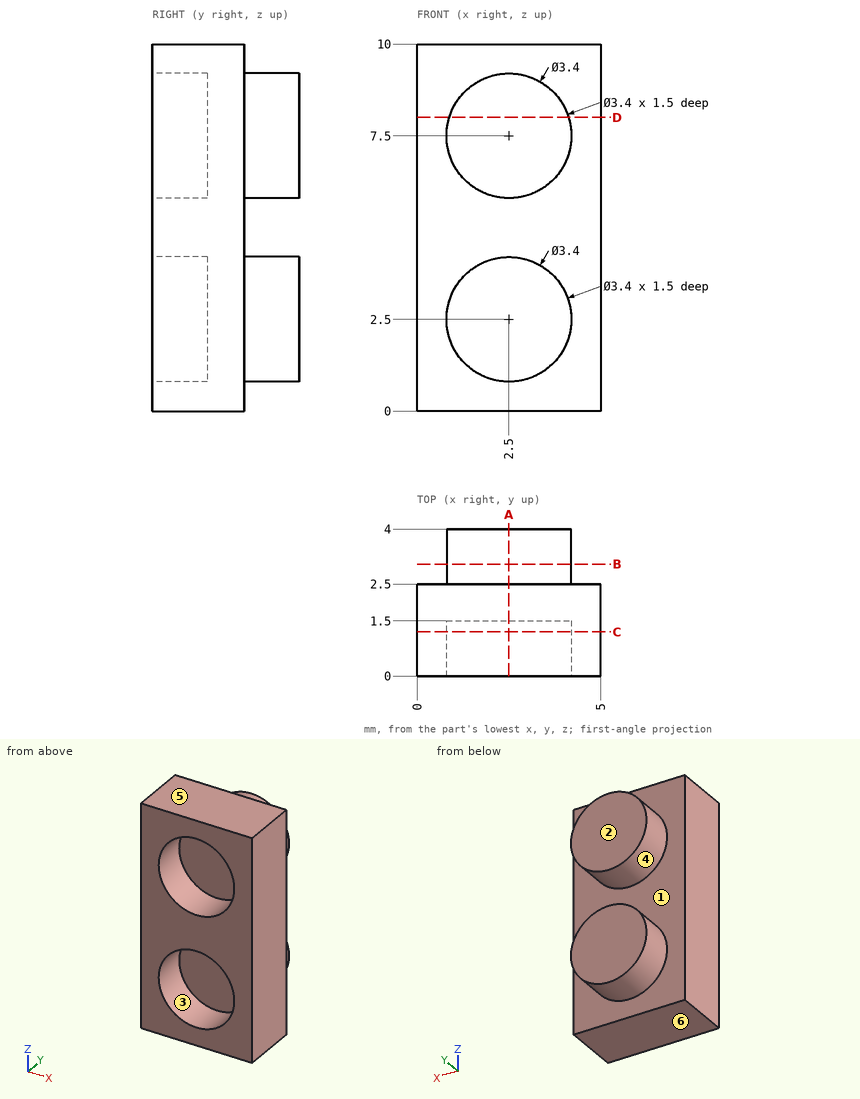
Verification items for this drawing (mm, ordinates from the low corner). A direction names the side the tool comes from. Round coordinates to 2 decimals unless told otherwise and drop trailing zeros. Order: outer loops, then holes, each group sorted by start corner. A loop starts at its lowest first (then second) coordinate and runs counter-clockwise, first axis right, second up. Notation, with made-up numbers: (69, 0.25) - (76, 0.25) arc R20 ccw to (76, 19.25) - close; hole circle Ø10 at (-37.5, 31). An arc over 180 degrees is marked (long way). Use CSV: the item, a comma, the result in double quotes. Start each with the question number.
1) Mould release check, pull along Z, two halves, no side actions. Record for the marked faces 4, 5 and 6: +Z half, -Z half, draft (parallel to the pull), parting line (faces both ways), or undercut.
2) Go/stop test with a flat-tipped pin: P1, Ø2, axis at x = 2.5, z = 8, coming from the -Y side. Record where the tip stops, or that it passes through.
3) Thickness scan on L1, parallel to Z at x = 2.5, y = 0.8; L2, parallel to Y at x = 1.75, z = 3.5; L3, parallel to Y at x = 4.5, z = 9.75. Record the ranges inside material, lowest first.
4) Access from +Z, -Z, +X, -X, +Y, -Y to the whole of each face (thin tool, end or side, straight path). Record for the marked faces 1, 2 and 3.
5) Section check D-D, the plane z = 8. Record the cut outline in (x, y).
6) Section check A-A, the plane x = 2.5. Record the cut outline in (y, z).
7) Section check C-C, the plane y = 1.2. Record the cut outline in (x, z), plus the area to 3 significant figures.
8) Section check B-B, the plane y = 3.05. Record the cut outline in (x, z), plus the area to 3 significant figures.
Answers:
1,face 4,"undercut"
1,face 5,"+Z half"
1,face 6,"-Z half"
2,P1,"stops at y = 1.5"
3,L1,"z = 0 to 0.8, 4.2 to 5.8, 9.2 to 10"
3,L2,"y = 1.5 to 4"
3,L3,"y = 0 to 2.5"
4,face 1,"+Y"
4,face 2,"+Z, -Z, +X, -X, +Y"
4,face 3,"-Y"
5,outline,"(0, 0) - (0.88, 0) - (0.88, 1.5) - (4.12, 1.5) - (4.12, 0) - (5, 0) - (5, 2.5) - (4.12, 2.5) - (4.12, 4) - (0.88, 4) - (0.88, 2.5) - (0, 2.5) - close"
6,outline,"(0, 0) - (2.5, 0) - (2.5, 0.8) - (4, 0.8) - (4, 4.2) - (2.5, 4.2) - (2.5, 5.8) - (4, 5.8) - (4, 9.2) - (2.5, 9.2) - (2.5, 10) - (0, 10) - (0, 9.2) - (1.5, 9.2) - (1.5, 5.8) - (0, 5.8) - (0, 4.2) - (1.5, 4.2) - (1.5, 0.8) - (0, 0.8) - close"
7,outline,"(0, 0) - (5, 0) - (5, 10) - (0, 10) - close; hole circle Ø3.4 at (2.5, 2.5); hole circle Ø3.4 at (2.5, 7.5)"
7,area,"31.8 mm²"
8,outline,"circle Ø3.4 at (2.5, 2.5); circle Ø3.4 at (2.5, 7.5)"
8,area,"18.2 mm²"
